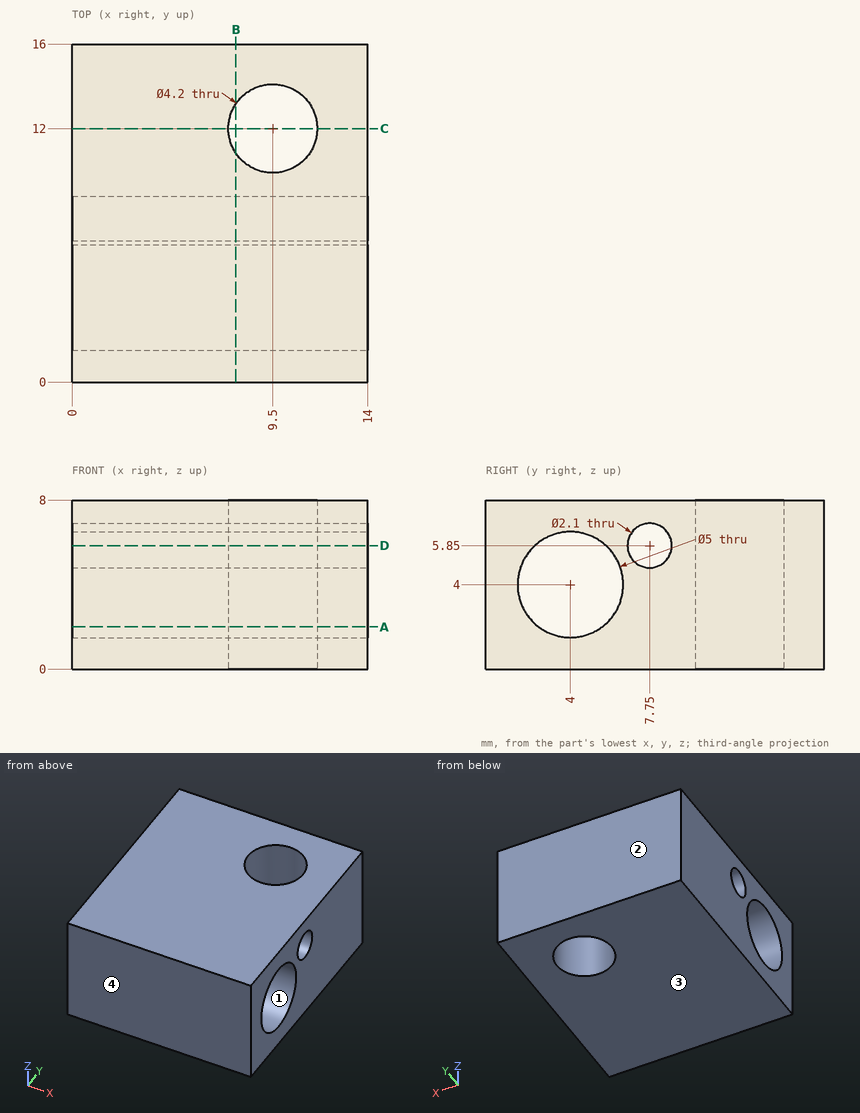
Input: dimensioned drawing with shaded views. Units: mm. Origin: part minimum x, y, z. Give positions to 0.01 mm unless a question says otherwise; leave off trailing zeros. Write each loop counter-clockwise with the first axis right and the second up, starting at its lowest first coordinate (ties: lowest second). Pieces come first, ordered by that corner, then holes.
1. Section query A-A (z = 2). Return the cut outline in (x, y), then the cut area to 3 significant figures.
2. Section query D-D (z = 5.85). Return the cut outline in (x, y), then the cut area to 3 significant figures.
3. First-contact query: pin 1 (2.5 mm diameter, centred on x = 9.5, y = 12, fed in from +Z). Flat tip, straight axial feed; report the tip coordinate or a pass-through.
4. Material intervals for line 1 along Y through (x, z) = (9.5, 4); line 2 along Y through (x, z) = (6, 5); line 3 along Y through (x, z) = (9.5, 6), sorted ascending.
5. Section query C-C (y = 12). Return the cut outline in (x, z), then the cut area to 3 significant figures.
6. Section query B-B (x = 7.75). Return the cut outline in (y, z).
7. Pull-direction query (Y, two-part tool) for the marked faces 1, 2, 3 and 4; classes: +Y half, -Y half, draft (parallel to the pull), parting line (faces both ways), or undercut.
Output values:
1. outline: (0, 0) - (14, 0) - (14, 2.5) - (0, 2.5) - close; (0, 5.5) - (14, 5.5) - (14, 16) - (0, 16) - close; hole circle Ø4.2 at (9.5, 12)
1. area: 168 mm2
2. outline: (0, 0) - (14, 0) - (14, 2.32) - (0, 2.32) - close; (0, 5.68) - (14, 5.68) - (14, 6.7) - (0, 6.7) - close; (0, 8.8) - (14, 8.8) - (14, 16) - (0, 16) - close; hole circle Ø4.2 at (9.5, 12)
2. area: 134 mm2
3. pin 1: passes through
4. line 1: y = 0 to 1.5, 6.5 to 9.9, 14.1 to 16
4. line 2: y = 0 to 1.71, 6.29 to 7.13, 8.37 to 16
4. line 3: y = 0 to 2.5, 5.5 to 6.71, 8.79 to 9.9, 14.1 to 16
5. outline: (0, 0) - (7.4, 0) - (7.4, 8) - (0, 8) - close; (11.6, 0) - (14, 0) - (14, 8) - (11.6, 8) - close
5. area: 78.4 mm2
6. outline: (0, 0) - (10.84, 0) - (10.84, 8) - (0, 8) - close; (13.16, 0) - (16, 0) - (16, 8) - (13.16, 8) - close; hole circle Ø5 at (4, 4); hole circle Ø2.1 at (7.75, 5.85)
7. face 1: undercut
7. face 2: +Y half
7. face 3: draft
7. face 4: -Y half
